```python
from build123d import *

# Parameters (mm, degrees)
F0_R           = 50.8
F0_R_2         = 25.4
F1_DEPTH       = 76.2
F2_DEPTH       = 152.4
F4_DEPTH       = 25.4
F6_D           = 25.4
F6_CSINK_D     = 50.8
F6_CSINK_ANGLE = 100


# Not quite as in the source:
# - a feature names something its author has since deleted; it is built from what else it names


with BuildPart() as f1:
    # F0 (on Top) → F1 (new body)
    with BuildSketch(Plane.XY):
        with BuildLine():
            Line((101.6, 203.2), (-101.6, 203.2))
            ThreePointArc((-101.6, 203.2), (-304.8, 0), (-101.6, -203.2))
            Line((-101.6, -203.2), (101.6, -203.2))
            ThreePointArc((101.6, -203.2), (304.8, 0), (101.6, 203.2))
        make_face()
        with BuildLine():
            ThreePointArc((-101.6, -127), (-228.6, 0), (-101.6, 127))
            Line((-101.6, 127), (101.6, 127))
            ThreePointArc((101.6, 127), (228.6, 0), (101.6, -127))
            Line((101.6, -127), (-101.6, -127))
        make_face(mode=Mode.SUBTRACT)
        with BuildLine():
            Line((101.6, 127), (-101.6, 127))
            ThreePointArc((-101.6, 127), (-228.6, 0), (-101.6, -127))
            Line((-101.6, -127), (101.6, -127))
            ThreePointArc((101.6, -127), (228.6, 0), (101.6, 127))
        make_face()
        with BuildLine():
            ThreePointArc((101.6, 63.5), (165.1, 0), (101.6, -63.5))
            Line((101.6, -63.5), (-101.6, -63.5))
            ThreePointArc((-101.6, -63.5), (-165.1, 0), (-101.6, 63.5))
            Line((-101.6, 63.5), (101.6, 63.5))
        make_face(mode=Mode.SUBTRACT)
        with BuildLine():
            Line((-101.6, -63.5), (101.6, -63.5))
            ThreePointArc((101.6, -63.5), (165.1, 0), (101.6, 63.5))
            Line((101.6, 63.5), (-101.6, 63.5))
            ThreePointArc((-101.6, 63.5), (-165.1, 0), (-101.6, -63.5))
        make_face()
        with Locations((-101.6, 0)):
            Circle(F0_R, mode=Mode.SUBTRACT)
        with Locations((101.6, 0)):
            Circle(F0_R, mode=Mode.SUBTRACT)
        with Locations((-101.6, 0)):
            Circle(F0_R)
        with Locations((-101.6, 0)):
            Circle(F0_R_2, mode=Mode.SUBTRACT)
        with Locations((101.6, 0)):
            Circle(F0_R)
        with Locations((101.6, 0)):
            Circle(F0_R_2, mode=Mode.SUBTRACT)
        with Locations((-101.6, 0)):
            Circle(F0_R_2)
        with Locations((101.6, 0)):
            Circle(F0_R_2)
    extrude(amount=F1_DEPTH)

    # F0 (on Top) → F2 (join)
    with BuildSketch(Plane.XY):
        with BuildLine():
            Line((101.6, 127), (-101.6, 127))
            ThreePointArc((-101.6, 127), (-228.6, 0), (-101.6, -127))
            Line((-101.6, -127), (101.6, -127))
            ThreePointArc((101.6, -127), (228.6, 0), (101.6, 127))
        make_face()
        with BuildLine():
            ThreePointArc((101.6, 63.5), (165.1, 0), (101.6, -63.5))
            Line((101.6, -63.5), (-101.6, -63.5))
            ThreePointArc((-101.6, -63.5), (-165.1, 0), (-101.6, 63.5))
            Line((-101.6, 63.5), (101.6, 63.5))
        make_face(mode=Mode.SUBTRACT)
        with Locations((101.6, 0)):
            Circle(F0_R)
        with Locations((101.6, 0)):
            Circle(F0_R_2, mode=Mode.SUBTRACT)
        with Locations((-101.6, 0)):
            Circle(F0_R)
        with Locations((-101.6, 0)):
            Circle(F0_R_2, mode=Mode.SUBTRACT)
        with Locations((101.6, 0)):
            Circle(F0_R_2)
        with Locations((-101.6, 0)):
            Circle(F0_R_2)
    extrude(amount=F2_DEPTH)

    # F3 (on face) → F4 (cut)
    with BuildSketch(Plane.XY):
        with BuildLine():
            Line((101.6, 101.6), (-101.6, 101.6))
            ThreePointArc((-101.6, 101.6), (-203.2, 0), (-101.6, -101.6))
            Line((-101.6, -101.6), (101.6, -101.6))
            ThreePointArc((101.6, -101.6), (203.2, 0), (101.6, 101.6))
        make_face()
    extrude(amount=F4_DEPTH, mode=Mode.SUBTRACT)

    # F6 (through all)
    with Locations(Plane.XY.offset(152.4)):
        with Locations((-101.6, 0), (101.6, 0)):
            CounterSinkHole(F6_D / 2, F6_CSINK_D / 2, counter_sink_angle=F6_CSINK_ANGLE)


solid = f1.part
```
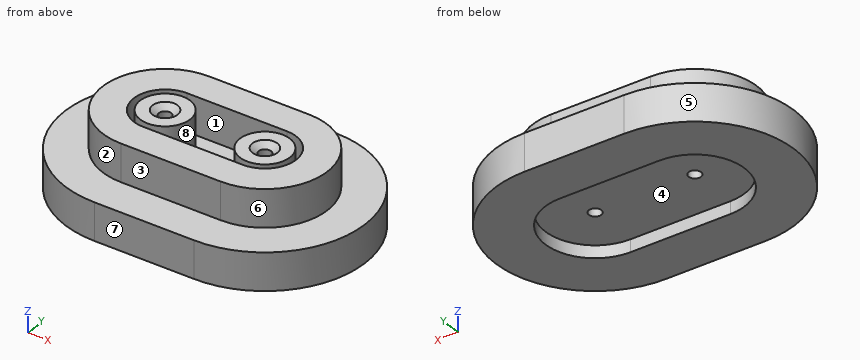
CAD build for the part. Positions are in the model's coordinates, mm. Face numbers are marked on the shaded views. A direction names the side the tool comes from. Coordinates: 2 decimals unless noted, no trailing zeros. Order: outer loops, then holes, each group sorted by start corner. A loop starts at its lowest first (then second) coordinate and runs counter-clockwise, first axis right, second up. Notation, with made-up numbers: (-0.5, 2.25) - (56.5, 2.25) arc R12 ccw to (56.5, 24.25) - close; hole circle Ø2 at (-20, 49.25). An arc over 180 degrees is marked (long way). Use a Markdown table: item, result. Add a question column.
(1) Which spindle directions (+Z, -Z, +X, -X, +Y, -Y) get a long thin tool onto all of the face, cutting with end or side? Do the marked faces 1, 2, 3 and 4. Say none if no direction does.
(2) Saw through at A-A (z = 103). Give the cut face in (x, y).
(3) Saw through at B-B (x = -37). Give the cut face in (y, z).
(4) Flat gauge pins, fed straight in: pin 1 (23 mm diameter, centred on x = 48, z = 108.5, fed in from -Y); pin 2 (6 mm diameter, centred on x = -111.5, y = 14, fed in from +Z); pin 3 (23 mm diameter, centred on x = -21.5, z = 105.5, fed in from +Y); pin 4 (5 mm diameter, centred on y = 131, z = 137, fed in from +X). Where does each tip first touch, or does it go through?
(5) Saw through at D-D (y = 0). Count the separate pieces of the cut face and the enclosed holes in it, then the cut area to 3 significant figures.
(6) Drill centre lines: line 1 along X through (y, z) = (0, 75); line 2 along Y through (x, z) = (-101, 105); line 3 along X through (y, z) = (0, 88). Where is each one in solid material? Low to high. Write a range as [from, to].
(7) Saw through at C-C (y = -75.5). Give the cut face in (x, z).
(8) Pull direction X, two halves, no side cores. Call the marked faces 5, 6, 7 and 8: +X half, -X half, draft (parallel to the pull), parting line (faces both ways), or undercut.
Solved:
| question | item | result |
|---|---|---|
| 1 | face 1 | +Z |
| 1 | face 2 | +Z, -X |
| 1 | face 3 | +Z, +X, -X, -Y |
| 1 | face 4 | -Z |
| 2 | outline | circle Ø101.6 at (-101.6, 0); (-101.6, -127) - (101.6, -127) arc R127 ccw to (101.6, 127) - (-101.6, 127) arc R127 ccw to start; circle Ø101.6 at (101.6, 0); hole circle Ø25.4 at (-101.6, 0); hole (-101.6, -63.5) - (101.6, -63.5) arc R63.5 ccw to (101.6, 63.5) - (-101.6, 63.5) arc R63.5 ccw to start; hole circle Ø25.4 at (101.6, 0) |
| 3 | outline | (-203.2, 0) - (-101.6, 0) - (-101.6, 25.4) - (101.6, 25.4) - (101.6, 0) - (203.2, 0) - (203.2, 76.2) - (127, 76.2) - (127, 152.4) - (63.5, 152.4) - (63.5, 76.2) - (-63.5, 76.2) - (-63.5, 152.4) - (-127, 152.4) - (-127, 76.2) - (-203.2, 76.2) - close |
| 4 | pin 1 | stops at y = -127 |
| 4 | pin 2 | stops at z = 147.99 |
| 4 | pin 3 | stops at y = 127 |
| 4 | pin 4 | passes through |
| 5 | separate pieces | 3 |
| 5 | enclosed holes | 0 |
| 5 | area | 54,600 mm² |
| 6 | line 1 | x = [-304.8, -114.3], [-88.9, 88.9], [114.3, 304.8] |
| 6 | line 2 | y = [-127, -63.5], [-50.8, -12.69], [12.69, 50.8], [63.5, 127] |
| 6 | line 3 | x = [-228.6, -165.1], [-152.4, -114.3], [-88.9, -50.8], [50.8, 88.9], [114.3, 152.4], [165.1, 228.6] |
| 7 | outline | (-290.25, 0) - (-169.59, 0) - (-169.59, 25.4) - (169.59, 25.4) - (169.59, 0) - (290.25, 0) - (290.25, 76.2) - (203.72, 76.2) - (203.72, 152.4) - (-203.72, 152.4) - (-203.72, 76.2) - (-290.25, 76.2) - close |
| 8 | face 5 | -X half |
| 8 | face 6 | +X half |
| 8 | face 7 | draft |
| 8 | face 8 | undercut |
